Geometry check sheet. Reference: the model listing, model coordinates, mm. A direction names the side the tool comes from. Give positions to 0.01 mm unless a question says otherwise; leave off trailing zeros. Write each loop counter-clockwise with the first axis right and the second up, starting at its lowest first coordinate (ties: lowest second). Pieces come first, ordered by that corner, then holes. Notation, with made-up numbers: (-5, 0) -> (22, 0) arc R30 ccw to (22, 24) -> close; hole circle Ø11 at (79, 18). An arc over 180 degrees is marked (long way). Write item = value, one per line. Start each with the question number.
1. Cross-section at B-B, the plane z = 0. Record the cut outline in (x, y).
2. Thickness scan on line 1 along X through (y, z) = (0.3, 0); line 2 along Y through (x, z) = (-30.5, -17.5); line 3 along Z through (x, y) = (22, 2). Record the ranges inside material, lowest first.
3. Depth check by flat-ended pin: P1, Ø1, axis at x = 4, y = 3.5, coming from the +Z side; P2, Ø2, axis at y = -1, z = -33.5, coming from the +X side; P3, Ø1.4, axis at x = -13, y = -1.5, coming from the -Z side; P4, Ø13, axis at x = 0, z = 0, coming from the +Y side. Enter the tip coordinate at first touch or a pass-through.
4. Set-up check for faces 1 (the flat face through (8, -1, 10)), 2 (the flat face through (-25, 1, -20)), 3 (the flat face through (0, 3, 17)), 4 (the flat face through (0, 1.75, -24)): record each of +Z, -Z, +X, -X, +Y, -Y from which the full face is reachable in a straight line by a thin tool's end or side.
5. Cross-section at D-D, the plane x = 16.5. Record the cut outline in (y, z), plus the area to 3 significant figures.
6. Cross-section at C-C, the plane y = -1.5. State how many separate pieces and enclosed holes the cut face has, plus the area to 3 significant figures.
7. Mould release check, pull along X, two halves, no side actions. Record for faces 5 (the cylindrical face through (11.06, -1.37, -30.7)), 6 (the flat face through (14.25, -1, 6)), 7 (the flat face through (-9, -1, 11.25)), 8 (the cylindrical face through (-10.61, -1.37, 6.76)): pulls with the +X half, pulls with the -X half, needs draft (parallel to the pull), parting line crosses it, or undercut.
8. Cross-section at A-A, the plane y = 3.5. Record the cut outline in (x, z).
```python
from build123d import *

# Parameters (mm, degrees)
BOSS_EXTRUDE1_DEPTH = 1.75
SKETCH2_W           = 70
SKETCH2_H           = 2
BOSS_EXTRUDE2_DEPTH = 3
SKETCH3_W           = 70
SKETCH3_H           = 4.2
BOSS_EXTRUDE3_DEPTH = 1.5
SKETCH4_W           = 6.25
SKETCH4_H           = 6.25
BOSS_EXTRUDE4_DEPTH = 2.7
SKETCH6_R           = 1.3
CUT_EXTRUDE2_DEPTH  = 51.474399452
FILLET3_R           = 3.5
SKETCH7_R           = 11
CUT_EXTRUDE3_DEPTH  = 50.877976102
CHAMFER1_SIZE       = 1.75
FILLET4_R           = 0.5


with BuildPart() as part:
    # Sketch1 → Boss-Extrude1 (new body)
    with BuildSketch(Plane(origin=(0, 0, 0), x_dir=(1, 0, 0), z_dir=(0, 1, 0))):
        Polygon((35, 20), (35, -20), (-35, -20), (-35, 20), (-14.25, 20), (-14.25, 35.25), (0, 35.25), (14.25, 35.25), (14.25, 20), align=None)
    extrude(amount=BOSS_EXTRUDE1_DEPTH)

    # Sketch2 → Boss-Extrude2 (add)
    with BuildSketch(Plane(origin=(0, 1.75, 0), x_dir=(1, 0, 0), z_dir=(0, 1, 0))):
        with Locations((0, 16)):
            Rectangle(SKETCH2_W, SKETCH2_H)
        with Locations((0, -16)):
            Rectangle(SKETCH2_W, SKETCH2_H)
    extrude(amount=BOSS_EXTRUDE2_DEPTH)

    # Sketch3 → Boss-Extrude3 (add)
    with BuildSketch(Plane(origin=(0, 4.75, 0), x_dir=(1, 0, 0), z_dir=(0, 1, 0))):
        with Locations((0, 17.1)):
            Rectangle(SKETCH3_W, SKETCH3_H)
        with Locations((0, -17.1)):
            Rectangle(SKETCH3_W, SKETCH3_H)
    extrude(amount=BOSS_EXTRUDE3_DEPTH)

    # Sketch4 → Boss-Extrude4 (add)
    with BuildSketch(Plane.XZ):
        Polygon((-11, -35.25), (-8, -35.25), (-8, -32), (-8, -29), (-11, -29), (-14.25, -29), (-14.25, -32), (-14.25, -35.25), align=None)
        with Locations((11.125, -32.125)):
            Rectangle(SKETCH4_W, SKETCH4_H)
        Polygon((14.25, 8), (14.25, 5), (8, 5), (8, 8.25), (8, 11.25), (14.25, 11.25), align=None)
        Polygon((-14.25, 11.25), (-8, 11.25), (-8, 8.25), (-8, 5), (-11, 5), (-14.25, 5), (-14.25, 8), align=None)
    extrude(amount=BOSS_EXTRUDE4_DEPTH)

    # Sketch6 → Cut-Extrude2 (cut, through all)
    with BuildSketch(Plane.XZ.offset(2.7)):
        with Locations(Location((-11, -32, 0), (0, 0, 270))):
            Circle(SKETCH6_R)
        with Locations(Location((11, -32, 0), (0, 0, 270))):
            Circle(SKETCH6_R)
        with Locations(Location((-11, 8, 0), (0, 0, 270))):
            Circle(SKETCH6_R)
        with Locations(Location((11, 8, 0), (0, 0, 270))):
            Circle(SKETCH6_R)
    extrude(amount=-CUT_EXTRUDE2_DEPTH, mode=Mode.SUBTRACT)

    # Fillet3
    fillet3_edges = [part.edges().sort_by_distance(p)[0] for p in [
        (-8, -1.35, 5),
        (-14.25, -1.35, 11.25),
        (8, -1.35, 5),
        (14.25, -1.35, 11.25),
        (-14.25, -0.475, -35.25),
        (14.25, -0.475, -35.25),
        (8, -1.35, -29),
        (-8, -1.35, -29),
    ]]
    fillet(fillet3_edges, radius=FILLET3_R)

    # Sketch7 → Cut-Extrude3 (cut, through all)
    with BuildSketch(Plane(origin=(0, 1.75, 0), x_dir=(1, 0, 0), z_dir=(0, 1, 0))):
        with Locations(Location((0, 0, 0), (0, 0, 270))):
            Circle(SKETCH7_R)
    extrude(amount=-CUT_EXTRUDE3_DEPTH, mode=Mode.SUBTRACT)

    # Chamfer1
    # the kernel refuses this chamfer: 1.75 mm, written as the material it takes off along each edge
    with BuildSketch(Plane(origin=(11, 1.75, -32), x_dir=(0, 0, -1), z_dir=(-1, 0, 0))) as chamfer1_piece_1:
        Polygon((1.3 + CHAMFER1_SIZE, 0), (1.3, CHAMFER1_SIZE), (1.3, 0), align=None)
    revolve(axis=Axis((11, 1.75, -32), (0, -1, 0)), mode=Mode.SUBTRACT)
    with BuildSketch(Plane(origin=(-11, 1.75, 8), x_dir=(0, 0, -1), z_dir=(-1, 0, 0))) as chamfer1_piece_2:
        Polygon((1.3 + CHAMFER1_SIZE, 0), (1.3, CHAMFER1_SIZE), (1.3, 0), align=None)
    revolve(axis=Axis((-11, 1.75, 8), (0, -1, 0)), mode=Mode.SUBTRACT)
    with BuildSketch(Plane(origin=(11, 1.75, 8), x_dir=(0, 0, -1), z_dir=(-1, 0, 0))) as chamfer1_piece_3:
        Polygon((1.3 + CHAMFER1_SIZE, 0), (1.3, CHAMFER1_SIZE), (1.3, 0), align=None)
    revolve(axis=Axis((11, 1.75, 8), (0, -1, 0)), mode=Mode.SUBTRACT)
    with BuildSketch(Plane(origin=(-11, 1.75, -32), x_dir=(0, 0, -1), z_dir=(-1, 0, 0))) as chamfer1_piece_4:
        Polygon((1.3 + CHAMFER1_SIZE, 0), (1.3, CHAMFER1_SIZE), (1.3, 0), align=None)
    revolve(axis=Axis((-11, 1.75, -32), (0, -1, 0)), mode=Mode.SUBTRACT)

    # Fillet4
    fillet4_edges = [part.edges().sort_by_distance(p)[0] for p in [
        (0, 4.75, -19.2),
        (0, 4.75, 19.2),
    ]]
    fillet(fillet4_edges, radius=FILLET4_R)


solid = part.part
```
Answers:
q1.outline = (-35, 0) -> (-11, 0) -> (-11, 1.75) -> (-35, 1.75) -> close; (11, 0) -> (35, 0) -> (35, 1.75) -> (11, 1.75) -> close
q2.line_1 = -35 to -11, 11 to 35
q2.line_2 = 0 to 1.75, 4.75 to 6.25
q2.line_3 = -17 to -15, 15 to 17
q3.P1 = 17
q3.P2 = 14.17
q3.P3 = -34.89
q3.P4 = through
q4.face_1 = +Z, -Z, -Y
q4.face_2 = -Z, -X, +Y, -Y
q4.face_3 = +Z, +X, -X
q4.face_4 = -Z, +X, -X
q5.outline = (0, -20) -> (1.75, -20) -> (1.75, -17) -> (4.75, -17) -> (4.75, -18.7) arc R0.5 ccw to (5.25, -19.2) -> (6.25, -19.2) -> (6.25, -15) -> (1.75, -15) -> (1.75, 15) -> (6.25, 15) -> (6.25, 19.2) -> (5.25, 19.2) arc R0.5 ccw to (4.75, 18.7) -> (4.75, 17) -> (1.75, 17) -> (1.75, 20) -> (0, 20) -> close
q5.area = 94.5 mm^2
q6.separate_pieces = 4
q6.enclosed_holes = 4
q6.area = 113 mm^2
q7.face_5 = undercut
q7.face_6 = pulls with the +X half
q7.face_7 = needs draft
q7.face_8 = undercut
q8.outline = (-35, -17) -> (35, -17) -> (35, -15) -> (-35, -15) -> close; (-35, 15) -> (35, 15) -> (35, 17) -> (-35, 17) -> close
